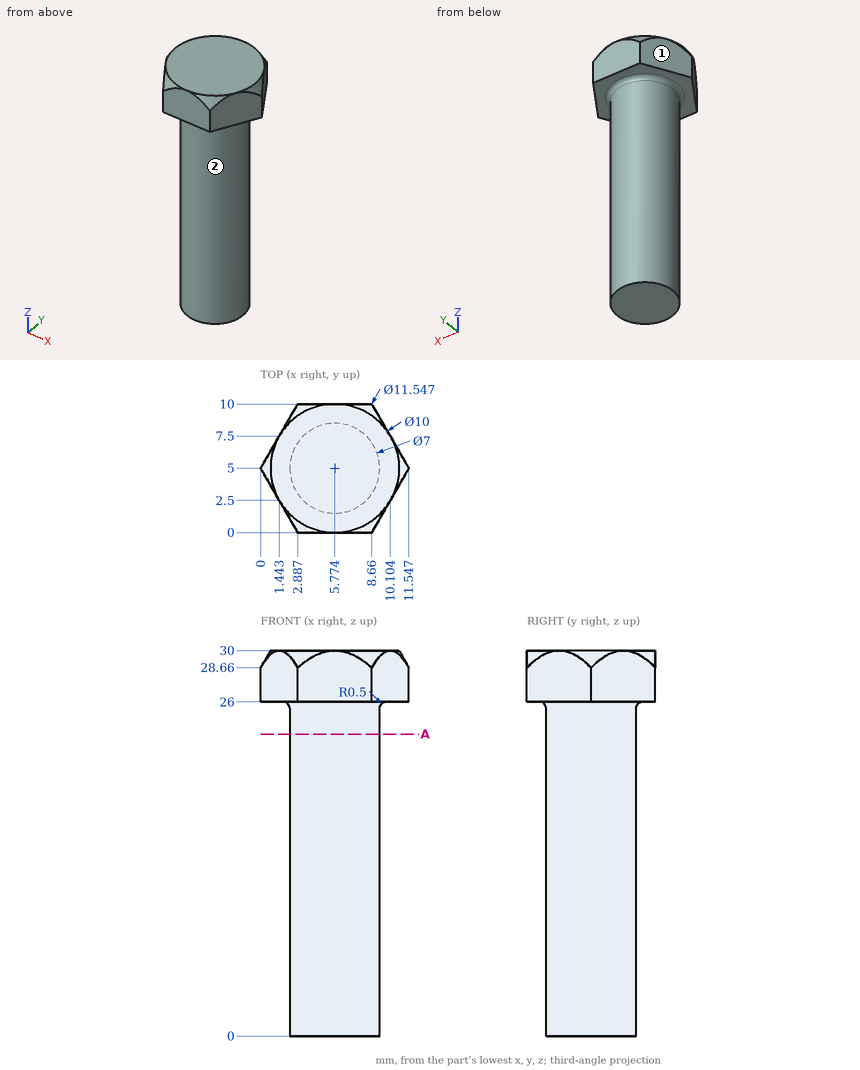
Geometry check sheet. Reference: drawing and pictorial views, mm from the part's lowest x, y, z. A direction names the side the tool comes from. Round coordinates to 2 decimals unless told otherwise and drop trailing zeros. Loops run counter-clockwise (first coordinate to the right, second up) from the corner with the lowest first, then second, coordinate; pieces in that order, holes last. Notation, with made-up numbers: M 37,31 L 49,31 A29 cw 49,65 Z; hole C -17,84 d10. An arc over 180 degrees is marked long. One line per item, written item: value.
(1) Depth check by flat-ended pin: pin 1 Ø3 at (y, z) = (6.5, 24) entering from -X; pin 2 Ø4 at (x, y) = (7, 1.5) entering from -Z; pin 3 Ø4 at (x, z) = (6, 5.5) entering from +Y; pin 4 Ø4 at (y, z) = (6, 18.5) entering from +X. Enter the tip coordinate at first touch or a pass-through.
Computed values:
pin 1: stops at x = 2.27
pin 2: stops at z = 0
pin 3: stops at y = 8.5
pin 4: stops at x = 9.27
(2) Thickness scan on line 1 (Z direction, x = 6.25, y = 9.75); line 2 (X direction, y = 3.5, z = 7) (1 decimal); line 3 (X direction, y = 7.5, z = 29) (1 decimal). Record the ranges inside material, lowest first.
Computed values:
line 1: z = 26 to 30
line 2: x = 2.6 to 8.9
line 3: x = 1.4 to 10.1
(3) Sectioned sample at A-A, the plane z = 23.5. Record the cut outline in (x, y).
Computed values:
outline: C 5.77,5 d7
(4) Access from +Z, -Z, +X, -X, +Y, -Y to the whole of each face (thin tool, end or side, straight path). Record for the marked faces 1 and 2.
Computed values:
face 1: +Z, -Z, -X, +Y
face 2: -Z
